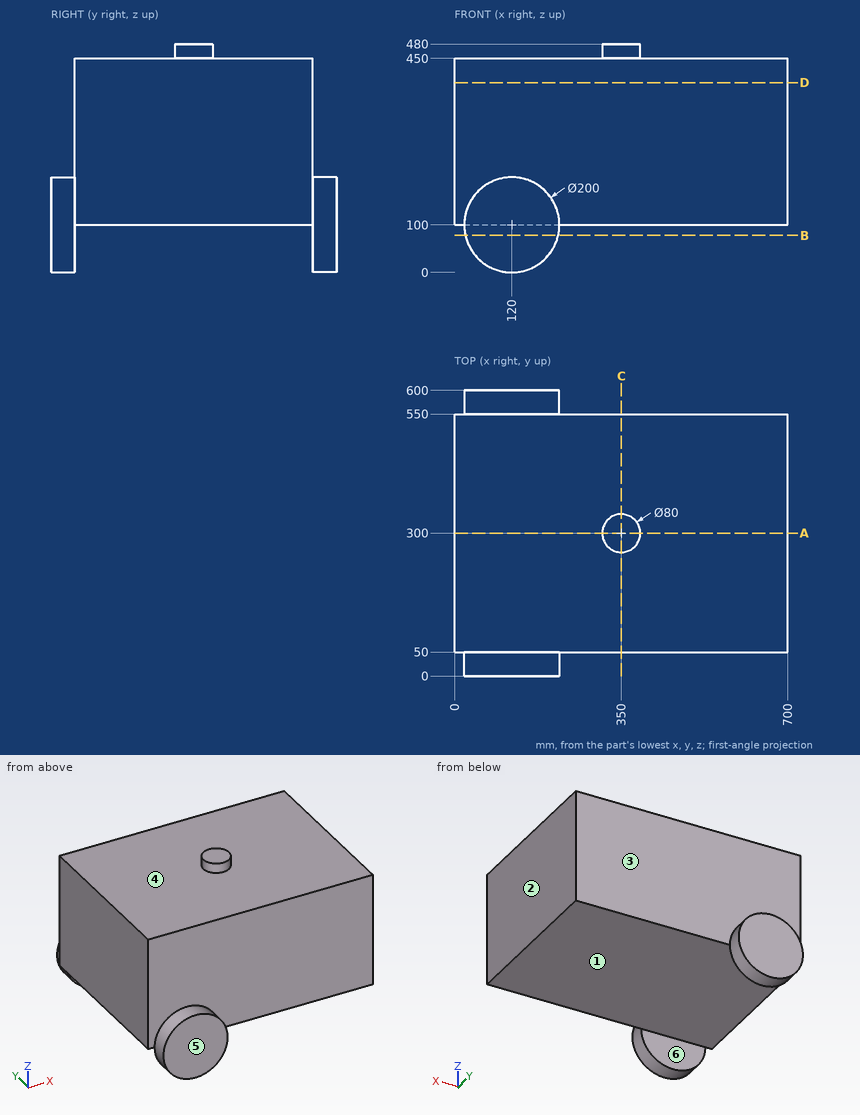
Geometry: see drawing. Coordinates: mm, zero at the bounding-box minimum. A direction names the side the tool comes from. Coordinates: 2 decimals unless noted, no trailing zeros. Loops run counter-clockwise (first coordinate to the right, second up) from the corner with the lowest first, then second, coordinate; pieces in that order, holes last.
Q1. Set-up query: the marked faces 1 and 2. Return all of +Z, -Z, +X, -X, +Y, -Y with unobstructed straight access to the full face (end or side cutting, diameter ignored); none if empty.
Q2. Cut plane D-D (z = 399). Output: boundary loops of the cut face in (x, y), then the cut area to 3 significant figures.
Q3. Contact query for flat-ended pins moving along their axis: pin 1 (1 mm diameter, centred on x = 101, y = 462, fed in from +Z); pin 2 (6 mm diameter, centred on y = 181, z = 342.5, fed in from -X); pin 3 (6 mm diameter, centred on x = 531.5, y = 183.5, fed in from -Z). Output: stop coordinate, or through.
Q4. Material intervals for line 1 (Z direction, x = 669, y = 332); line 2 (Y direction, x = 269, z = 226.5); line 3 (X direction, y = 557.5, z = 131), sorted ascending.
Q5. Cut plane B-B (z = 78). Output: boundary loops of the cut face in (x, y).
Q6. Draft query along Y for the marked faces 3, 4, 5 and 6. Return one class per face: +Y half, -Y half, draft (parallel to the pull), parting line (faces both ways), or undercut.
Q7. Cut plane A-A (y = 300). Output: boundary loops of the cut face in (x, z), then the cut area to 3 significant figures.
Q8. Cut plane C-C (x = 350). Output: boundary loops of the cut face in (y, z).
Working result:
1. face 1: -Z, +X, -X
1. face 2: +Z, -Z, +X, +Y, -Y
2. outline: (0, 50) - (700, 50) - (700, 550) - (0, 550) - close
2. area: 350,000 mm2
3. pin 1: stops at z = 450
3. pin 2: stops at x = 0
3. pin 3: stops at z = 100
4. line 1: z = 100 to 450
4. line 2: y = 50 to 550
4. line 3: x = 24.93 to 215.07
5. outline: (22.45, 0) - (217.55, 0) - (217.55, 50) - (22.45, 50) - close; (22.45, 550) - (217.55, 550) - (217.55, 600) - (22.45, 600) - close
6. face 3: +Y half
6. face 4: draft
6. face 5: -Y half
6. face 6: undercut
7. outline: (0, 100) - (700, 100) - (700, 450) - (390, 450) - (390, 480) - (310, 480) - (310, 450) - (0, 450) - close
7. area: 247,000 mm2
8. outline: (50, 100) - (550, 100) - (550, 450) - (340, 450) - (340, 480) - (260, 480) - (260, 450) - (50, 450) - close
